Part model, mm, in its own coordinate system. Give positions to 0.01 mm unless a question says otherwise; leave off trailing zeros. Loops run counter-clockwise (first coordinate to the right, second up) from the corner with the lowest first, then second, coordinate; pieces in that order, holes last. Notation, with made-up numbers: M -15,76.25 L -3,76.25 A19 cw -3,90.25 Z; hole C 23.5,81.25 d7. An arc over 180 degrees is marked long. Answer in a Markdown table with one row per item.
from build123d import *

# Parameters (mm, degrees)
BOSS_EXTRUDE1_DEPTH = 44.45
FILLET1_R           = 0.127
CHAMFER2_SIZE       = 1.27


with BuildPart() as part:
    # Sketch1 → Boss-Extrude1 (new body)
    with BuildSketch(Plane.XY):
        Polygon((0, 0), (0, 86.36), (8.89, 0), align=None)
    extrude(amount=BOSS_EXTRUDE1_DEPTH)

    # Fillet1
    fillet1_edges = [part.edges().sort_by_distance(p)[0] for p in [
        (0, 86.36, 22.225),
    ]]
    fillet(fillet1_edges, radius=FILLET1_R)

    # Chamfer2
    # the kernel refuses this chamfer: 1.27 mm, written as the material it takes off along each edge
    with BuildSketch(Plane(origin=(0, -3.266037395, 0), x_dir=(0, 0, 1), z_dir=(0, 1, 0))) as chamfer2_piece_1:
        Polygon((CHAMFER2_SIZE, 0), (0, CHAMFER2_SIZE), (0, 0), align=None)
    extrude(amount=90.418126679, mode=Mode.SUBTRACT)
    with BuildSketch(Plane(origin=(0, 0, -3.266037395), x_dir=(0, 1, 0), z_dir=(0, 0, 1))) as chamfer2_piece_2:
        Polygon((CHAMFER2_SIZE, 0), (0, -CHAMFER2_SIZE), (0, 0), align=None)
    extrude(amount=50.982074789, mode=Mode.SUBTRACT)
    with BuildSketch(Plane(origin=(0, -3.266037395, 44.45), x_dir=(0, 0, -1), z_dir=(0, 1, 0))) as chamfer2_piece_3:
        Polygon((CHAMFER2_SIZE, 0), (0, -CHAMFER2_SIZE), (0, 0), align=None)
    extrude(amount=90.418126679, mode=Mode.SUBTRACT)


solid = part.part
(1) Saw through at A-A (z = 12). Write the cut outline in (x, y).
Recorded:
| item | result |
|---|---|
| outline | M 0,1.27 L 1.27,0 L 8.89,0 L 0.25,83.9 A0.13 ccw 0,83.89 Z |
(2) Saw through at B-B (y = 14). Write the cut outline in (x, z).
Recorded:
| item | result |
|---|---|
| outline | M 0,1.27 L 1.27,0 L 7.45,0 L 7.45,44.45 L 1.27,44.45 L 0,43.18 Z |
(3) Saw through at C-C (x = 6). Write the cut outline in (y, z), plus the area to 3 significant figures.
Recorded:
| item | result |
|---|---|
| outline | M 0,0 L 28.07,0 L 28.07,44.45 L 0,44.45 Z |
| area | 1,250 mm^2 |
(4) Saw through at D-D (y = 32.5). Write the cut outline in (x, z), plus the area to 3 significant figures.
Recorded:
| item | result |
|---|---|
| outline | M 0,1.27 L 1.27,0 L 5.54,0 L 5.54,44.45 L 1.27,44.45 L 0,43.18 Z |
| area | 245 mm^2 |
(5) Drill centre lines: line 1 along Z through (x, y) = (1.25, 36.5); line 2 along X through (y, z) = (13.5, 31); line 3 along X through (y, z) = (50, 16). Where is each one in solid material? Low to high.
Recorded:
| item | result |
|---|---|
| line 1 | z = 0.02 to 44.43 |
| line 2 | x = 0 to 7.5 |
| line 3 | x = 0 to 3.74 |
(6) Pin check, flat tips, straight feed: pin 1 Ø1.5 at (y, z) = (69.5, 32.5) entering from +X; pin 2 Ø3 at (x, z) = (1, 15.5) entering from +Y; pin 3 Ø5 at (x, y) = (6, 73.5) entering from -Z. Stop position of each tip, or through.
Recorded:
| item | result |
|---|---|
| pin 1 | stops at x = 1.81 |
| pin 2 | stops at y = 84.01 |
| pin 3 | passes through |
